from build123d import *

# Parameters (mm, degrees)
F0_R     = 8
F0_R_2   = 6
F1_DEPTH = 8
F2_DEPTH = 7
F3_R     = 8
F3_R_2   = 6
F3_R_3   = 2.5
F4_DEPTH = 1
F5_DEPTH = 15.001


# Not quite as in the source:
# - a feature names something its author has since deleted; it is built from what else it names


with BuildPart() as f1:
    # F0 (on Top) → F1 (new body)
    with BuildSketch(Plane.XY):
        Circle(F0_R)
        Circle(F0_R_2, mode=Mode.SUBTRACT)
        Circle(F0_R_2)
    extrude(amount=F1_DEPTH)

    # F0 (on Top) → F2 (join)
    with BuildSketch(Plane.XY):
        Circle(F0_R_2)
    extrude(amount=-F2_DEPTH)

    # F3 (on face) → F4 (join)
    with BuildSketch(Plane(origin=(0, 0, -7), x_dir=(1, 0, 0), z_dir=(0, 0, -1))):
        Circle(F3_R)
        Circle(F3_R_2, mode=Mode.SUBTRACT)
        Circle(F3_R_2)
        Circle(F3_R_3, mode=Mode.SUBTRACT)
    extrude(amount=F4_DEPTH)

    # F3 (on face) → F5 (cut, through all)
    with BuildSketch(Plane(origin=(0, 0, -7), x_dir=(1, 0, 0), z_dir=(0, 0, -1))):
        Circle(F3_R_3)
    extrude(amount=-F5_DEPTH, mode=Mode.SUBTRACT)


solid = f1.part
Could you check a few things on this model? Use its own coordinates, in mm. A direction names the side the tool comes from. Give positions to 0.01 mm unless a question says otherwise; leave off trailing zeros. Loops run counter-clockwise (first coordinate to the right, second up) from the corner with the lowest first, then second, coordinate; pieces in that order, holes last. Notation, with made-up numbers: (-13, -13.5) -> (15, -13.5) arc R11 ccw to (15, 4.5) -> close; hole circle Ø6 at (50, 70). An arc over 180 degrees is marked (long way). Answer as CSV lines item,"result". Start each with the question number.
(1) If we section it at A-A on y = 0: Write out the boundary of the cut face in (x, z).
(2) I'm going to push flat-ended pins straight in: pin 1 Ø3 at (x, z) = (-6, -4) entering from -Y; pin 2 Ø2 at (y, z) = (2, 1) entering from +X; pin 3 Ø4.5 at (x, y) = (0, 0) entering from -Z; pin 4 Ø4 at (y, z) = (1, -4.5) entering from +X. Where does each tip first touch, or does it pass through?
(3) If we section it at C-C on z = 7: Write out the boundary of the cut face in (x, y), then the cut area to 3 significant figures.
(4) We'd pull the mould along Z, two halves only. Please class faces 3 (the cylindrical face through (-1.73, 7.81, -7.49)), 4 (the cylindrical face through (-6, 0, -3)), 5 (the flat face through (2, -2, -8)): released by +Z, released by -Z, zero draft, split by the parting line, or undercut.
(5) I need wall thicknesses on probe 1 along Y at (x, z) = (0, 1); probe 2 along Z at (x, y) = (-1, -6). Which ranges of each line are inside material? Lowest first, please.
(6) Which directions (+Z, -Z, +X, -X, +Y, -Y) give clear straight access to the entire face, cutting with the end or side of a thin tool? Please do faces 1 (the flat face through (-2, -6, -7)), 2 (the cylindrical face through (-1.73, -7.81, 3.94)).
(7) If we section it at D-D on y = -4.75: Write out the boundary of the cut face in (x, z), then the cut area to 3 significant figures.
Computed:
1,outline,"(-8, -8) -> (-2.5, -8) -> (-2.5, 8) -> (-8, 8) -> (-8, 0) -> (-6, 0) -> (-6, -7) -> (-8, -7) -> close; (2.5, -8) -> (8, -8) -> (8, -7) -> (6, -7) -> (6, 0) -> (8, 0) -> (8, 8) -> (2.5, 8) -> close"
2,pin 1,"stops at y = -3.97"
2,pin 2,"stops at x = 7.94"
2,pin 3,"passes through"
2,pin 4,"stops at x = 6"
3,outline,"circle Ø16 at (0, 0); hole circle Ø5 at (0, 0)"
3,area,"181 mm2"
4,face 3,"zero draft"
4,face 4,"undercut"
4,face 5,"released by -Z"
5,probe 1,"y = -8 to -2.5, 2.5 to 8"
5,probe 2,"z = -8 to -7, 0 to 8"
6,face 1,"none"
6,face 2,"+Z, -Z"
7,outline,"(-6.44, -8) -> (6.44, -8) -> (6.44, -7) -> (3.67, -7) -> (3.67, 0) -> (6.44, 0) -> (6.44, 8) -> (-6.44, 8) -> (-6.44, 0) -> (-3.67, 0) -> (-3.67, -7) -> (-6.44, -7) -> close"
7,area,"167 mm2"
